Geometry check sheet. Reference: the model listing, model coordinates, mm. A direction names the side the tool comes from. Round coordinates to 2 decimals unless told otherwise and drop trailing zeros. Order: outer loops, then holes, each group sorted by start corner. A loop starts at its lowest first (then second) coordinate and runs counter-clockwise, first axis right, second up. Notation, with made-up numbers: (84.5, 53.5) -> (99.5, 53.5) arc R24 ccw to (99.5, 69.5) -> close; hole circle Ø10 at (-6.75, -26.75). An arc over 180 degrees is marked (long way). Use a Markdown table: item, result. Add a question column.
Item 1: Sectioned sample at A-A, the plane z = 22. Record the cut outline in (x, y).
Item 2: Sectioned sample at B-B, the plane x = 62. Record the cut outline in (y, z), and give its area (3 significant figures).
Item 3: Sectioned sample at C-C, the plane y = 16. Record the cut outline in (x, z), and give its area (3 significant figures).
Item 4: Mould release check, pull along Y, two halves, no side actions. Record for faces 4 (the flat face through (39, 0, 0)), 5 (the flat face through (-46, -11, 7)), 6 (the flat face through (-46, -13, 7)): pulls with the +Y half, pulls with the -Y half, needs draft (parallel to the pull), parting line crosses it, or undercut.
Item 5: Sectioned sample at D-D, the plane x = 0. Record the cut outline in (y, z).
Item 6: Material ranges on probe 1 along Y at (x, z) = (45, 66); probe 2 along Z at (x, y) = (-2.5, -9.5); probe 3 along X at (y, z) = (0, 71), recorded low to high. Write a range as [from, to].
Item 7: Gauge pin test, flat ends, axial feed: pin 1 Ø1 at (x, y) = (27.5, -21) entering from +Z; pin 2 Ø4 at (x, z) = (68.5, 78) entering from +Y; pin 3 Ø15.5 at (x, z) = (-43, 8.5) entering from -Y. Record the tip position at first contact, or that the pin passes through.
Item 8: Set-up check for faces 1 (the cylindrical face through (17.535, -33.713, 190.874)), 2 (the flat face through (48, 32, 54)), 3 (the flat face through (48, -32, 54)): record each of +Z, -Z, +X, -X, +Y, -Y from which the full face is reachable in a straight line by a thin tool's end or side.
from build123d import *
from build123d.topology import SkipClean

# Parameters (mm, degrees)
SKETCH1_R                      = 40
SKETCH1_R_2                    = 38
BOSS_EXTRUDE1_DEPTH            = 200
SKETCH2_R                      = 40
BOSS_EXTRUDE2_DEPTH            = 2
BOSS_EXTRUDE3_DEPTH            = 107
BOSS_EXTRUDE4_DEPTH            = 2
SKETCH5_R                      = 1.75
CUT_EXTRUDE1_DEPTH             = 225.428162226
CUT_EXTRUDE2_REACH             = 218.296
SKETCH6_R                      = 4
CUT_EXTRUDE2_DIRECTION_2_REACH = 218.296
CIRPATTERN1_COUNT              = 2
CIRPATTERN1_ANGLE              = 90
BOSS_EXTRUDE5_REACH            = 241.742
BOSS_EXTRUDE5_END_RADIUS       = 40
SKETCH7_W                      = 14
SKETCH7_H                      = 2
CUT_EXTRUDE3_REACH             = 221.073
SKETCH8_R                      = 1.75
FILLET1_R                      = 3
CUT_EXTRUDE4_REACH             = 220.598
SKETCH9_R                      = 0.25
BOSS_EXTRUDE6_START            = 2
BOSS_EXTRUDE6_DEPTH            = 2


with BuildPart() as part:
    # Sketch1 → Boss-Extrude1 (new body)
    with BuildSketch(Plane.XY):
        Circle(SKETCH1_R)
        Circle(SKETCH1_R_2, mode=Mode.SUBTRACT)
    extrude(amount=BOSS_EXTRUDE1_DEPTH)

    # Sketch2 → Boss-Extrude2 (add)
    with BuildSketch(Plane.XY.offset(180)):
        Circle(SKETCH2_R)
    extrude(amount=BOSS_EXTRUDE2_DEPTH)

    # Sketch3 → Boss-Extrude3 (add)
    with BuildSketch(Plane(origin=(0, 0, 0), x_dir=(-1, 0, 0), z_dir=(0, 0, -1))):
        with BuildLine():
            Line((-24, -32), (-72, -32))
            Line((-72, -32), (-72, -30))
            Line((-72, -30), (-26.457513111, -30))
            ThreePointArc((-26.457513111, -30), (-25.248567431, -31.024342744), (-24, -32))
        make_face()
        with BuildLine():
            Line((-24, 32), (-72, 32))
            Line((-72, 32), (-72, 30))
            Line((-72, 30), (-26.457513111, 30))
            ThreePointArc((-26.457513111, 30), (-25.248567431, 31.024342744), (-24, 32))
        make_face()
    extrude(amount=-BOSS_EXTRUDE3_DEPTH)

    # Sketch4 → Boss-Extrude4 (add)
    with BuildSketch(Plane.XY.offset(107)):
        with BuildLine():
            Line((72, -32), (24, -32))
            ThreePointArc((24, -32), (40, 0), (24, 32))
            Line((24, 32), (72, 32))
            Line((72, 32), (72, -32))
        make_face()
    extrude(amount=BOSS_EXTRUDE4_DEPTH)

    # Sketch5 → Cut-Extrude1 (cut, through all)
    with BuildSketch(Plane(origin=(0, 32, 0), x_dir=(1, 0, 0), z_dir=(0, 1, 0))):
        with Locations(Location((43.5, -102.5, 0), (0, 0, 270))):
            Circle(SKETCH5_R)
        with Locations(Location((43.5, -3.5, 0), (0, 0, 270))):
            Circle(SKETCH5_R)
        with Locations(Location((68.5, -78, 0), (0, 0, 270))):
            Circle(SKETCH5_R)
    extrude(amount=-CUT_EXTRUDE1_DEPTH, mode=Mode.SUBTRACT)

    # Sketch6 → Cut-Extrude2 (cut, up to next)
    with BuildSketch(Plane(origin=(0, 0, 0), x_dir=(0, 0, 1), z_dir=(-0.7071067811865488, 0.7071067811865464, 0)), mode=Mode.PRIVATE) as cut_extrude2_sk1:
        with Locations(Location((187, 0, 0), (0, 0, 90))):
            Circle(SKETCH6_R)
    cut_extrude2_tool1 = extrude(cut_extrude2_sk1.sketch, amount=-CUT_EXTRUDE2_REACH, mode=Mode.PRIVATE) & part.part
    cut_extrude2 = cut_extrude2_tool1.solids().sort_by_distance((0, 0, 187))[0]
    add(cut_extrude2, mode=Mode.SUBTRACT)

    # Sketch6 → Cut-Extrude2 direction 2 (cut, up to next)
    with BuildSketch(Plane(origin=(0, 0, 0), x_dir=(0, 0, 1), z_dir=(-0.7071067811865488, 0.7071067811865464, 0)), mode=Mode.PRIVATE) as cut_extrude2_direction_2_sk1:
        with Locations(Location((187, 0, 0), (0, 0, 90))):
            Circle(SKETCH6_R)
    cut_extrude2_direction_2_tool1 = extrude(cut_extrude2_direction_2_sk1.sketch, amount=CUT_EXTRUDE2_DIRECTION_2_REACH, mode=Mode.PRIVATE) & part.part
    cut_extrude2_direction_2 = cut_extrude2_direction_2_tool1.solids().sort_by_distance((0, 0, 187))[0]
    add(cut_extrude2_direction_2, mode=Mode.SUBTRACT)

    # CirPattern1: Cut-Extrude2, Cut-Extrude2 direction 2 ×2 about axis
    cirpattern1_axis = Axis((0, 0, -12.1), (0, 0, 1))
    add([cut_extrude2.rotate(cirpattern1_axis, i * CIRPATTERN1_ANGLE / (CIRPATTERN1_COUNT - 1)) for i in range(1, CIRPATTERN1_COUNT)], mode=Mode.SUBTRACT)
    add([cut_extrude2_direction_2.rotate(cirpattern1_axis, i * CIRPATTERN1_ANGLE / (CIRPATTERN1_COUNT - 1)) for i in range(1, CIRPATTERN1_COUNT)], mode=Mode.SUBTRACT)

    # Boss-Extrude5: up to this cylinder (the profile starts outside it)
    boss_extrude5_end = Plane(origin=(0, 0, 7), z_dir=(0, 0, -1)) * Cylinder(BOSS_EXTRUDE5_END_RADIUS, 564.484, mode=Mode.PRIVATE)
    # Sketch7 → Boss-Extrude5 (add, up to the surface)
    with BuildSketch(Plane(origin=(-54, 0, 0), x_dir=(0, 0, -1), z_dir=(1, 0, 0)), mode=Mode.PRIVATE) as boss_extrude5_sk1:
        with Locations((-7, -12)):
            Rectangle(SKETCH7_W, SKETCH7_H)
    boss_extrude5_tool1 = extrude(boss_extrude5_sk1.sketch, amount=BOSS_EXTRUDE5_REACH, mode=Mode.PRIVATE) - boss_extrude5_end
    add(boss_extrude5_tool1.solids().sort_by_distance((-54, -12, 7))[0])
    # Sketch7 → Boss-Extrude5 (add, up to the surface)
    with BuildSketch(Plane(origin=(-54, 0, 0), x_dir=(0, 0, -1), z_dir=(1, 0, 0)), mode=Mode.PRIVATE) as boss_extrude5_sk2:
        with Locations((-7, 12)):
            Rectangle(SKETCH7_W, SKETCH7_H)
    boss_extrude5_tool2 = extrude(boss_extrude5_sk2.sketch, amount=BOSS_EXTRUDE5_REACH, mode=Mode.PRIVATE) - boss_extrude5_end
    add(boss_extrude5_tool2.solids().sort_by_distance((-54, 12, 7))[0])

    # Cut-Extrude3: up to this face of the body (flat: up to its plane)
    cut_extrude3_end = Plane(part.part.faces().sort_by_distance((-45.914280319, 13, 7))[0])
    # Sketch8 → Cut-Extrude3 (cut, up to the picked face)
    with BuildSketch(Plane.XZ.offset(13), mode=Mode.PRIVATE) as cut_extrude3_sk1:
        with Locations(Location((-49.770305539, 5.008755099, 0), (0, 0, 270))):
            Circle(SKETCH8_R)
    cut_extrude3_tool1 = split(extrude(cut_extrude3_sk1.sketch, amount=-CUT_EXTRUDE3_REACH, mode=Mode.PRIVATE), bisect_by=cut_extrude3_end, keep=Keep.BOTH, mode=Mode.PRIVATE)
    add(cut_extrude3_tool1.solids().sort_by(Axis((-49.770306, -13, 5.008755), (0, 1, 0)))[0], mode=Mode.SUBTRACT)

    # Fillet1
    fillet1_edges = [part.edges().sort_by_distance(p)[0] for p in [
        (-54, -12, 14),
        (-54, -12, 0),
        (-54, 12, 0),
        (-54, 12, 14),
    ]]
    fillet(fillet1_edges, radius=FILLET1_R)

    # Sketch9 → Cut-Extrude4 (cut, up to next)
    with BuildSketch(Plane.XZ.offset(-11), mode=Mode.PRIVATE) as cut_extrude4_sk1:
        with Locations(Location((-43.770305539, 7.008755099, 0), (0, 0, 270))):
            Circle(SKETCH9_R)
    cut_extrude4_tool1 = extrude(cut_extrude4_sk1.sketch, amount=-CUT_EXTRUDE4_REACH, mode=Mode.PRIVATE) & part.part
    add(cut_extrude4_tool1.solids().sort_by_distance((-43.770306, 11, 7.008755))[0], mode=Mode.SUBTRACT)

    # Sketch10 → Boss-Extrude6 (add)
    with SkipClean():  # the faces are left unmerged after this step: merging them gives an invalid solid
        with BuildSketch(Plane(origin=(0, 0, 0), x_dir=(-1, 0, 0), z_dir=(0, 0, -1)).offset(BOSS_EXTRUDE6_START)):
            with BuildLine():
                ThreePointArc((10, -36.66060556), (0, -38), (-10, -36.66060556))
                Line((-10, -36.66060556), (-10, -38.729833462))
                ThreePointArc((-10, -38.729833462), (0, -40), (10, -38.729833462))
                Line((10, -38.729833462), (10, -36.66060556))
            make_face()
            with BuildLine():
                ThreePointArc((10, 38.729833462), (0, 40), (-10, 38.729833462))
                Line((-10, 38.729833462), (-10, 36.66060556))
                ThreePointArc((-10, 36.66060556), (0, 38), (10, 36.66060556))
                Line((10, 36.66060556), (10, 38.729833462))
            make_face()
        extrude(amount=-BOSS_EXTRUDE6_DEPTH)


solid = part.part
Found:
| question | item | result |
|---|---|---|
| 1 | outline | (24, -32) -> (72, -32) -> (72, -30) -> (26.46, -30) arc R40 ccw to (26.46, 30) -> (72, 30) -> (72, 32) -> (24, 32) arc R40 ccw (long way) to start; hole circle Ø76 at (0, 0) |
| 2 | outline | (-32, 0) -> (-30, 0) -> (-30, 107) -> (30, 107) -> (30, 0) -> (32, 0) -> (32, 109) -> (-32, 109) -> close |
| 2 | area | 556 mm2 |
| 3 | outline | (-36.66, 0) -> (-34.47, 0) -> (-34.47, 180) -> (34.47, 180) -> (34.47, 0) -> (36.66, 0) -> (36.66, 107) -> (72, 107) -> (72, 109) -> (36.66, 109) -> (36.66, 200) -> (34.47, 200) -> (34.47, 182) -> (-34.47, 182) -> (-34.47, 200) -> (-36.66, 200) -> close |
| 3 | area | 1,090 mm2 |
| 4 | face 4 | needs draft |
| 4 | face 5 | undercut |
| 4 | face 6 | pulls with the -Y half |
| 5 | outline | (-40, -2) -> (-38, -2) -> (-38, 180) -> (38, 180) -> (38, -2) -> (40, -2) -> (40, 200) -> (38, 200) -> (38, 182) -> (-38, 182) -> (-38, 200) -> (-40, 200) -> close |
| 6 | probe 1 | y = [-32, -30], [30, 32] |
| 6 | probe 2 | z = [180, 182] |
| 6 | probe 3 | x = [-40, -38], [38, 40] |
| 7 | pin 1 | stops at z = 182 |
| 7 | pin 2 | stops at y = 32 |
| 7 | pin 3 | stops at y = -18.91 |
| 8 | face 1 | +Z |
| 8 | face 2 | +Z, -Z, +X, +Y |
| 8 | face 3 | +Z, -Z, +X, -Y |
